from build123d import *

# Parameters (mm, degrees)
SM_BASE_FLANGE_1_DEPTH  = 30
FILLET_1_R              = 30
SKETCH_2_R              = 4.75
CUT_EXTRUDE_1_DEPTH     = 10
HOLE_WIZARD_1_OUTLINE_R = 1.6
HOLE_WIZARD_1_DEPTH     = 5
SKETCH_5_R              = 10
CUT_EXTRUDE_2_DEPTH     = 10
HOLE_WIZARD_2_OUTLINE_R = 1.6
HOLE_WIZARD_2_DEPTH     = 5


# Read off the part's stored shape, not the designer's step: 孔1, 孔2
# Sheet-metal steps are written as plain solids
with BuildPart() as part:
    # Sketch 1 → 基体-法兰1 (new, symmetric)
    with BuildSketch(Plane.XY):
        with BuildLine():
            Line((60, 0), (5.7366, 0))
            ThreePointArc((5.7366, 0), (1.680211239, 1.680211239), (0, 5.7366))
            Line((0, 5.7366), (0, 104))
            Line((0, 104), (5, 104))
            Line((5, 104), (5, 5.7366))
            ThreePointArc((5, 5.7366), (5.215745145, 5.215745145), (5.7366, 5))
            Line((5.7366, 5), (60, 5))
            Line((60, 5), (60, 0))
        make_face()
    extrude(amount=SM_BASE_FLANGE_1_DEPTH, both=True)

    # 圆角1
    fillet_1_edges = [part.edges().sort_by_distance(p)[0] for p in [
        (60, 2.5, -30),
        (60, 2.5, 30),
        (2.5, 104, -30),
        (2.5, 104, 30),
    ]]
    fillet(fillet_1_edges, radius=FILLET_1_R - 0.0001)  # a hair under: the kernel refuses the full size

    # Sketch 2 → 切除-拉伸1 (cut)
    with BuildSketch(Plane(origin=(0, 5, 0), x_dir=(1, 0, 0), z_dir=(0, 1, 0))):
        with Locations(Location((30, 0, 0), (0, 0, 180))):
            Circle(SKETCH_2_R)
    extrude(amount=-CUT_EXTRUDE_1_DEPTH, mode=Mode.SUBTRACT)

    # 孔1 outline → 孔1 (cut)
    with BuildSketch(Plane(origin=(0, 0, 0), x_dir=(1, 0, 0), z_dir=(0, 1, 0))):
        with Locations((23.25, -11.691342951)):
            Circle(HOLE_WIZARD_1_OUTLINE_R)
        with Locations((16.5, 0)):
            Circle(HOLE_WIZARD_1_OUTLINE_R)
        with Locations((23.25, 11.691342951)):
            Circle(HOLE_WIZARD_1_OUTLINE_R)
        with Locations((36.75, 11.691342951)):
            Circle(HOLE_WIZARD_1_OUTLINE_R)
        with Locations((43.5, 0)):
            Circle(HOLE_WIZARD_1_OUTLINE_R)
        with Locations((36.75, -11.691342951)):
            Circle(HOLE_WIZARD_1_OUTLINE_R)
    extrude(amount=HOLE_WIZARD_1_DEPTH, mode=Mode.SUBTRACT)

    # 草图5 → 切除-拉伸2 (cut)
    with BuildSketch(Plane.ZY):
        with Locations(Location((0, 74, 0), (0, 0, 270))):
            Circle(SKETCH_5_R)
    extrude(amount=-CUT_EXTRUDE_2_DEPTH, mode=Mode.SUBTRACT)

    # 孔2 outline → 孔2 (cut)
    with BuildSketch(Plane.YZ):
        with Locations((60.564971157, 13.435028843)):
            Circle(HOLE_WIZARD_2_OUTLINE_R)
        with Locations((60.564971157, -13.435028843)):
            Circle(HOLE_WIZARD_2_OUTLINE_R)
        with Locations((87.435028843, -13.435028843)):
            Circle(HOLE_WIZARD_2_OUTLINE_R)
        with Locations((87.435028843, 13.435028843)):
            Circle(HOLE_WIZARD_2_OUTLINE_R)
    extrude(amount=HOLE_WIZARD_2_DEPTH, mode=Mode.SUBTRACT)


solid = part.part
Build history of the part. All positions in model axes, mm. A direction names the side the tool comes from. Coordinates: 2 decimals unless noted, no trailing zeros. Write each loop counter-clockwise with the first axis right and the second up, starting at its lowest first coordinate (ties: lowest second). Pieces come first, ordered by that corner, then holes. Notation, with made-up numbers: (-26, -24) -> (20, -24) arc R20 cw to (20, 5) -> close; hole circle Ø8 at (51, 58). An arc over 180 degrees is marked (long way). Use CSV: the item, a comma, the result in double quotes. Start each with the question number.
Q1. Cut at A-A, the plane x = 23.25. List the corners of the cut face in (y, z).
Q2. 3-axis set-ups, long thin cutter, end or side, ignore diameter. For faces 1 (the flat face through (32, 5, 7)), 2 (the cylindrical face through (24.776, 2.465, -12.172)): which of +Z, -Z, +X, -X, +Y, -Y reach the whole face in a straight line?
Q3. Cut at B-B, the plane y = 65.5. List the corners of the cut face in (x, z).
Q4. Cut at C-C, the plane z = -8. List the corners of the cut face in (x, y).
Q5. Drill centre lines: probe 1 along Z at (x, y) = (23, 1); probe 2 along X at (y, z) = (8, 24). Where is each one in solid material? Low to high.
Q6. Pull direction Y, two halves, no side cores. Call faces 3 (the cylindrical face through (2, 84, 0)), 4 (the cylindrical face through (1.725, 1.636, 0.42)), 5 (the cylindrical face through (2.46, 62.09, 13.92)), 6 (the cylindrical face through (37.49, 2.46, 13.11)): released by +Y, released by -Y, zero draft, split by the parting line, or undercut.
Q7. Flat gauge pins, fed straight in: pin 1 Ø18 at (y, z) = (35.5, -5) entering from +X; pin 2 Ø5 at (x, z) = (47.5, 21) entering from +Y. Where does each tip first touch, or does it go through?
Q8. Cut at D-D, the plane x = 16.5. List the corners of the cut face in (y, z), then the cut area to 3 significant figures.
Checked values:
1,outline,"(0, -30) -> (5, -30) -> (5, -13.29) -> (0, -13.29) -> close; (0, -10.09) -> (5, -10.09) -> (5, 10.09) -> (0, 10.09) -> close; (0, 13.29) -> (5, 13.29) -> (5, 30) -> (0, 30) -> close"
2,face 1,"+Z, -Z, +X, +Y"
2,face 2,"+Y, -Y"
3,outline,"(0, -30) -> (5, -30) -> (5, -5.27) -> (0, -5.27) -> close; (0, 5.27) -> (5, 5.27) -> (5, 30) -> (0, 30) -> close"
4,outline,"(0, 5.74) arc R5.74 ccw to (5.74, 0) -> (58.91, 0) -> (58.91, 5) -> (5.74, 5) arc R0.74 cw to (5, 5.74) -> (5, 68) -> (0, 68) -> close; (0, 80) -> (5, 80) -> (5, 102.91) -> (0, 102.91) -> close"
5,probe 1,"z = -30 to -13.27, -10.11 to 10.11, 13.27 to 30"
5,probe 2,"x = 0 to 5"
6,face 3,"undercut"
6,face 4,"released by -Y"
6,face 5,"undercut"
6,face 6,"zero draft"
7,pin 1,"stops at x = 5"
7,pin 2,"stops at y = 5"
8,outline,"(0, -30) -> (5, -30) -> (5, -1.6) -> (0, -1.6) -> close; (0, 1.6) -> (5, 1.6) -> (5, 30) -> (0, 30) -> close"
8,area,"284 mm²"
